Part model, mm, in its own coordinate system. Face numbers are marked on the shaded views. A direction names the side the tool comes from. Round coordinates to 2 decimals unless told otherwise and drop trailing zeros. Write each loop counter-clockwise with the first axis right and the second up, starting at its lowest first coordinate (ties: lowest second). Pieces come first, ordered by that corner, then holes. Notation, with made-up numbers: M 86,69 L 103,69 A5 ccw 103,74 Z; hole C 46.5,87.25 d5. An arc over 180 degrees is marked long. Use one line per item in the form item = value. Start each with the question number.
Item 1: Probe L1, parallel to Z at x = -4.5, y = 3.05; L2, parallel to Z at x = -9, y = 5; L3, parallel to Y at x = -3.65, z = -3. List the from-to ranges inside material, lowest first.
Item 2: Mould opens along X. For the marked faces 4, 5 and 6 say: +X half, -X half, draft (parallel to the pull), parting line (faces both ways), or undercut.
Item 3: Flat gauge pins, fed straight in: pin 1 Ø1 at (y, z) = (1, -5.5) entering from +X; pin 2 Ø0.8 at (y, z) = (2.5, -2.5) entering from +X. Where does each tip first touch, or does it go through?
Item 4: Cut at C-C, the plane y = 2.65. Give the cut face in (x, z).
Item 5: Cut at B-B, the plane x = -9.25. Give the cut face in (y, z), then the cut area to 3 significant figures.
Item 6: Cut at D-D, the plane x = -1. Give the cut face in (y, z).
Item 7: Which spindle directions (+Z, -Z, +X, -X, +Y, -Y) get a long thin tool onto all of the face, cutting with end or side? Do the marked faces 1, 2 and 3. Say none if no direction does.
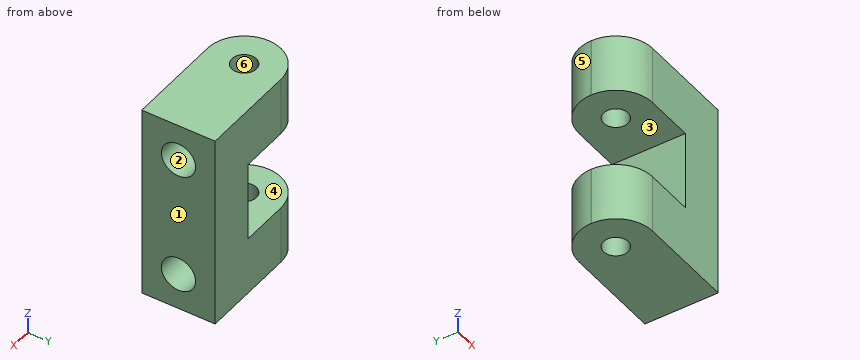
Autodesk Inventor part; units mm, degrees
ref_plane "YZ Plane" through (0, 0, 0) normal (1, 0, 0) x (0, 1, 0)
ref_plane "XZ Plane" through (0, 0, 0) normal (0, 1, 0) x (-1, 0, 0)
ref_plane "XY Plane" through (0, 0, 0) normal (0, 0, 1) x (1, 0, 0)
sketch "Sketch7" plane through (0, 0, 0) normal (0, 1, 0) x (-1, 0, 0)
  line L0 (0, 0) -> (0, -16)
  line L1 (0, -16) -> (11, -16)
  line L2 (11, -16) -> (11, -11.25)
  line L3 (11, -11.25) -> (4, -11.25)
  line L4 (4, -11.25) -> (4, -4.75)
  line L5 (4, -4.75) -> (11, -4.75)
  line L6 (11, -4.75) -> (11, 0)
  line L7 (11, 0) -> (0, 0)
  dimension "d25" = 16
  dimension "d26" = 6.5
  dimension "d27" = 7
  dimension "d28" = 4
extrude "Extrusion7" add sketch "Sketch7" along normal blind 6
sketch "Sketch8" plane through (0, 0, 0) normal (1, 0, 0) x (0, 0, -1)
  line L0 (0, 0) -> (16, 0)
  line L1 (16, 0) -> (16, 6)
  line L2 (16, 6) -> (0, 6)
  line L3 (0, 0) -> (0, 6)
  line L4 (4.75, 6) -> (11.25, 6) construction
  line L5 (8, 6) -> (8, 0) construction
  line L6 (11.25, 0) -> (4.75, 0) construction
  line L7 (16, 0) -> (16, 6) construction
  line L8 (16, 3) -> (0, 3) construction
  line L9 (0, 0) -> (0, 6) construction
  circle A0 centre (3, 3) radius 1.4
  circle A1 centre (13, 3) radius 1.4
  dimension "d31" = 2.8
  dimension "d32" = 10
extrude "Extrusion8" cut sketch "Sketch8" against normal blind 6 contours A0 | A1
sketch "Sketch9" plane through (-11, 0, 0) normal (0, 0, 1) x (1, 0, 0)
  line L0 (0, 0) -> (11, 0)
  line L1 (11, 0) -> (11, 6)
  line L2 (11, 6) -> (0, 6)
  line L3 (0, 0) -> (0, 6)
  line L4 (11, 0) -> (11, 6) construction
  line L5 (11, 3) -> (0, 3) construction
  circle A0 centre (3, 3) radius 1
  dimension "d35" = 2
  dimension "d36" = 3
extrude "Extrusion9" cut sketch "Sketch9" against normal through all contours A0
fillet "Fillet2" radius 3 4 edges at (-11, 6, -13.625) (-11, 0, -13.625) (-11, 6, -2.375) (-11, 0, -2.375)
properties part number "drzak_pritlaku"
Model answer:
q1.L1 = -16 to -14.4, -11.6 to -11.25, -4.75 to -4.4, -1.6 to 0
q1.L2 = -16 to -11.25, -4.75 to 0
q1.L3 = 0 to 1.6, 4.4 to 6
q2.face_4 = draft
q2.face_5 = -X half
q2.face_6 = undercut
q3.pin_1 = 0
q3.pin_2 = -6
q4.outline = M -10.98,-16 L -8.94,-16 L -8.94,-11.25 L -10.98,-11.25 Z; M -10.98,-4.75 L -8.94,-4.75 L -8.94,0 L -10.98,0 Z; M -7.06,-16 L 0,-16 L 0,-14.36 L -6,-14.36 L -6,-11.64 L 0,-11.64 L 0,-4.36 L -6,-4.36 L -6,-1.64 L 0,-1.64 L 0,0 L -7.06,0 L -7.06,-4.75 L -4,-4.75 L -4,-11.25 L -7.06,-11.25 Z
q5.outline = M 0.27,-16 L 5.73,-16 L 5.73,-11.25 L 0.27,-11.25 Z; M 0.27,-4.75 L 5.73,-4.75 L 5.73,0 L 0.27,0 Z
q5.area = 51.8 mm²
q6.outline = M 0,-16 L 6,-16 L 6,0 L 0,0 Z; hole C 3,-13 d2.8; hole C 3,-3 d2.8
q7.face_1 = +Z, -Z, +X, +Y, -Y
q7.face_2 = +X
q7.face_3 = -X, +Y, -Y
